Autodesk Inventor part; units mm, degrees
ref_plane "YZ Plane" through (0, 0, 0) normal (1, 0, 0) x (0, 1, 0)
ref_plane "XZ Plane" through (0, 0, 0) normal (0, 1, 0) x (-1, 0, 0)
ref_plane "XY Plane" through (0, 0, 0) normal (0, 0, 1) x (1, 0, 0)
sketch "Sketch1" plane through (0, 0, 0) normal (0, 1, 0) x (-1, 0, 0)
  line L0 (0, 0) -> (161, 0)
  line L1 (161, 0) -> (161, -115)
  line L2 (161, -115) -> (0, -115)
  line L3 (0, -115) -> (0, 0)
  dimension "d0" = 161
  dimension "d1" = 115
extrude "Extrusion1" add sketch "Sketch1" along normal blind 56
fillet "Fillet1" radius 2.5 12 edges at (0, 56, -57.5) (0, 28, -115) (0, 28, 0) (0, 0, -57.5) (-80.5, 0, 0) (-80.5, 0, -115) (-80.5, 56, -115) (-80.5, 56, 0) (-161, 56, -57.5) (-161, 28, 0) (-161, 28, -115) (-161, 0, -57.5)
sketch "Sketch2" plane through (0, 2.5, -112.5) normal (1, 0, 0) x (0, 0, -1)
  line L0 (2.5, 0) -> (2.5, 51)
  line L1 (0, 0) -> (-110, 0)
  line L2 (0, 51) -> (0, 0)
  line L3 (-110, 51) -> (0, 51)
  line L4 (-110, 0) -> (-110, 51)
  line L5 (0, 53.5) -> (-110, 53.5)
  line L6 (-41.5, 29) -> (-27.5, 29)
  line L7 (-27.5, 29) -> (-27.5, 22)
  line L8 (-27.5, 22) -> (-41.5, 22)
  line L9 (-41.5, 22) -> (-41.5, 29)
  line L10 (-85, 30) -> (-67.5, 30)
  line L11 (-67.5, 30) -> (-67.5, 25)
  line L12 (-67.5, 25) -> (-85, 25)
  line L13 (-85, 25) -> (-85, 30)
  circle A0 centre (-30.5, 25.5) radius 2
  line L14 (-41.5, 22.5) -> (-35.5, 22.5)
  line L15 (-35.5, 22.5) -> (-35.5, 28.5)
  line L16 (-35.5, 28.5) -> (-41.5, 28.5)
  line L17 (-41.5, 28.5) -> (-41.5, 22.5)
  line L18 (-41.5, 22.5) -> (-35.5, 28.5) construction
  line L19 (-35.5, 22.5) -> (-41.5, 28.5) construction
  circle A1 centre (-16.5, 25.5) radius 7
  circle A2 centre (-16.5, 27.5) radius 3
  point P0 (-112.5, -2.5)
  point P1 (-38.5, 25.5)
  point P2 (-41.5, 22.5)
  dimension "d5" = 26
  dimension "d6" = 19
  dimension "d7" = 14
  dimension "d8" = 7
  dimension "d9" = 30
  dimension "d10" = 17.5
  dimension "d11" = 5
  dimension "d12" = 70
  dimension "d13" = 23.5
  dimension "d14" = 24.5
  dimension "d15" = 4
  dimension "d16" = 33
  dimension "d17" = 41
  dimension "d18" = 6
  dimension "d19" = 6
  dimension "d20" = 14
  dimension "d21" = 19
  dimension "d22" = 6
  dimension "d44" = 28
  dimension "d45" = 28
  dimension "d46" = 28
extrude "Extrusion2" cut sketch "Sketch2" against normal blind 10 contours A2
extrude "Extrusion3" cut sketch "Sketch2" against normal blind 0.1 contours A1
extrude "Extrusion4" cut sketch "Sketch2" against normal blind 10 contours A0
extrude "Extrusion5" cut sketch "Sketch2" against normal blind 5 contours L6 L7 L8 L9 L14 L15 L16 | L16 L15 L14 L9 | A0
extrude "Extrusion7" cut sketch "Sketch2" against normal blind 0.2 contours L10 L11 L12 L13
sketch "Sketch3" plane through (-10, 30, -96) normal (1, 0, 0) x (0, 0, -1)
  circle A0 centre (0, 0) radius 1.25
  point P0 (-96, -30)
  dimension "d35" = 2.5
extrude "Extrusion8" add sketch "Sketch3" along normal blind 8
fillet "Fillet2" radius 1.25 1 edges at (-2, 30, -94.75)
sketch "Sketch4" plane through (-5, 2.5, -112.5) normal (1, 0, 0) x (0, 0, -1)
  circle A0 centre (-38.5, 25.5) radius 1.4
  circle A1 centre (-38.5, 25.5) radius 0.9
  point P0 (-112.5, -2.5)
  dimension "d39" = 2.8
  dimension "d40" = 1.8
extrude "Extrusion9" add sketch "Sketch4" along normal blind 5
fillet "Fillet3" radius 0.25 2 edges at (0, 28, -73.1) (0, 28, -72.6)
properties part number "22Ah BatteryPack"
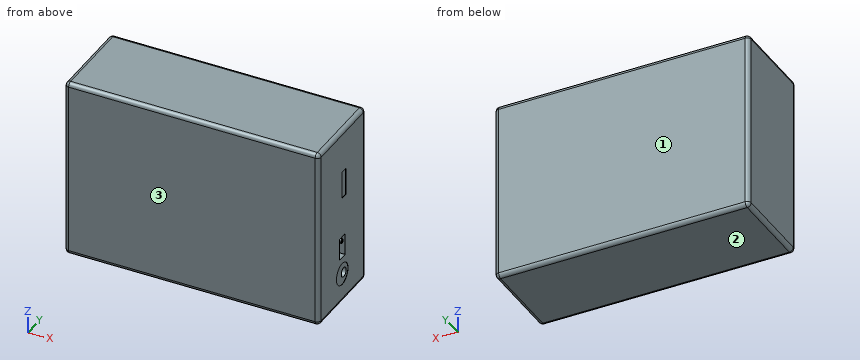
Can you work these out from the model? Positions are in its coordinate system, mm. Face numbers are marked on the shaded views. Coordinates: 2 decimals unless noted, no trailing zeros. Return JSON: item names as keys, results as strings.
Q1. Please list where these lines run through material, in increasing order: L1, parallel to Y at x = -4, z = -96; L2, parallel to Y at x = -2, z = -74. Write a range as from..to.
Computed values:
{"L1": "y = 0..27, 28.75..31.25, 33..56", "L2": "y = 0.05..24.5, 26.6..27.1, 28.9..29.4, 31.5..55.95"}
Q2. I'm going to push flat-ended pins straight in: pin 1 Ø6 at (y, z) = (39.5, -87.5) entering from +X; pin 2 Ø1.4 at (y, z) = (28, -74) entering from +X; pin 3 Ø3 at (y, z) = (29.5, -97) entering from +X; pin 4 Ø2.5 at (y, z) = (29, -40) entering from +X. Where does each tip first touch, or does it pass through?
Computed values:
{"pin 1": "stops at x = 0", "pin 2": "stops at x = -5", "pin 3": "stops at x = -2", "pin 4": "stops at x = -0.2"}
Q3. Thinking about a two-plate mould opening in Y: for the marked faces 1, 2 and 3, which applies, +Y half, -Y half, draft (parallel to the pull), parting line (faces both ways), or undercut?
Computed values:
{"face 1": "+Y half", "face 2": "draft", "face 3": "-Y half"}
